Geometry check sheet. Reference: the model listing, model coordinates, mm. Coordinates: 2 decimals unless noted, no trailing zeros. Write each loop counter-clockwise with the first axis right and the second up, starting at its lowest first coordinate (ties: lowest second). Pieces come first, ordered by that corner, then holes. Notation, with made-up numbers: (-15.75, -31.75) -> (31.25, -31.75) arc R21 ccw to (31.25, 3.25) -> close; hole circle Ø7 at (50.25, 47.5). An arc over 180 degrees is marked (long way). One line per question, with ' | ' between items.
Autodesk Inventor part; units mm, degrees
ref_plane "YZ Plane" through (0, 0, 0) normal (1, 0, 0) x (0, 1, 0)
ref_plane "XZ Plane" through (0, 0, 0) normal (0, 1, 0) x (-1, 0, 0)
ref_plane "XY Plane" through (0, 0, 0) normal (0, 0, 1) x (1, 0, 0)
sketch "Sketch1" plane through (0, 0, 0) normal (0, 0, 1) x (1, 0, 0)
  arc A0 (5.0089, -4.6844) -> (-5.0089, -4.6844) centre (0, 0) ccw
  line L0 (0, 0) -> (0, 3.3219)
  line L1 (0, 0) -> (0, -6.858)
  line L2 (4.1269, 0.3611) -> (4.5966, 0.4021)
  line L3 (-4.1269, 0.3611) -> (-4.5966, 0.4021)
  line L4 (-3.0829, -2.3997) -> (-3.5588, -4.3082)
  line L5 (3.0829, -2.3997) -> (3.5588, -4.3082)
  arc A1 (0.8337, 3.4569) -> (-0.8337, 3.4569) centre (0, 0) ccw
  arc A2 (-3.5485, -0.2304) -> (-3.1723, -1.6067) centre (0, 0) ccw
  arc A3 (3.1723, -1.6067) -> (3.5485, -0.2304) centre (0, 0) ccw
  arc A4 (3.5588, -4.3082) -> (5.0089, -4.6844) centre (4.3861, -4.102) ccw
  arc A5 (-5.0089, -4.6844) -> (-3.5588, -4.3082) centre (-4.3861, -4.102) ccw
  arc A6 (4.1269, 0.3611) -> (3.5485, -0.2304) centre (4.1822, -0.2715) ccw
  arc A7 (3.1723, -1.6067) -> (3.0829, -2.3997) centre (4.192, -2.1232) ccw
  arc A8 (-3.5485, -0.2304) -> (-4.1269, 0.3611) centre (-4.1822, -0.2715) ccw
  arc A9 (-3.0829, -2.3997) -> (-3.1723, -1.6067) centre (-4.192, -2.1232) ccw
  arc A10 (4.5966, 0.4021) -> (5.3741, 1.5314) centre (4.5191, 1.2878) ccw
  arc A11 (3.0157, 4.7044) -> (1.3489, 4.3144) centre (2.3718, 3.6998) ccw
  arc A12 (-5.3741, 1.5314) -> (-4.5966, 0.4021) centre (-4.5191, 1.2878) ccw
  arc A13 (-1.3489, 4.3144) -> (-3.0157, 4.7044) centre (-2.3718, 3.6998) ccw
  line L6 (-0.8337, 3.4569) -> (-1.3489, 4.3144)
  line L7 (0.8337, 3.4569) -> (1.3489, 4.3144)
  arc A14 (5.3741, 1.5314) -> (3.0157, 4.7044) centre (0, 0) ccw
  arc A15 (-3.0157, 4.7044) -> (-5.3741, 1.5314) centre (0, 0) ccw
  point P0 (5.5667, 0.487)
  point P1 (-5.5667, 0.487)
  point P2 (-3.7479, -5.1854)
  point P3 (2.9716, -1.9532)
  point P4 (3.7479, -5.1854)
  point P5 (1.4868, 5.1225)
  point P6 (0, 2.4453)
  point P7 (-1.4868, 5.1225)
  point P8 (0, 2.4453)
  point P9 (-2.9716, -1.9532)
  point P10 (-0.8419, 3.4705)
  point P11 (-2.3046, 5.9049)
  point P12 (0.8419, 3.4705)
  point P13 (2.3046, 5.9049)
  dimension "d0" = 13.716
  dimension "d2" = 95
  dimension "d3" = 14
  dimension "d4" = 3.556
  dimension "d5" = 0.8527
  dimension "d6" = 3.556
  dimension "d7" = 14
  dimension "d8" = 1.27
  dimension "d9" = 1.27
  dimension "d10" = 1.778
  dimension "d11" = 31
  dimension "d12" = 2.286
extrude "Extrusion1" add sketch "Sketch1" along normal blind 0.6858
equation "\"d6\" = d4"
equation "\"d7\" = d3"
equation "\"d9\" = d8"
properties material "Steel"
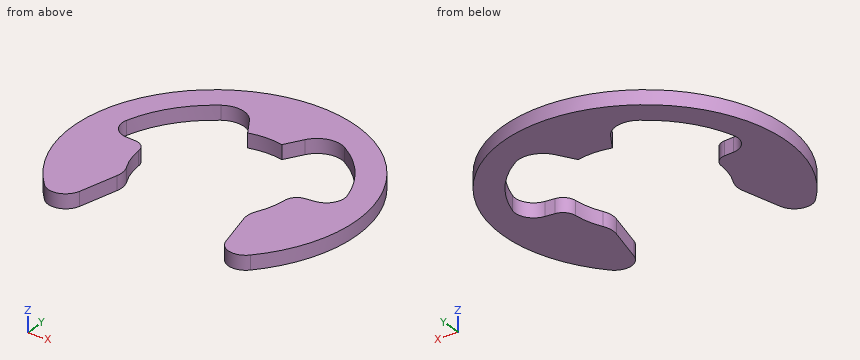
1. Cross-section at C-C on x = 4.75. Record the boundary of the cut face in (y, z).
Worked answers:
outline: (-4.87, 0) -> (0.43, 0) -> (0.43, 0.69) -> (-4.87, 0.69) -> close; (2.94, 0) -> (4.95, 0) -> (4.95, 0.69) -> (2.94, 0.69) -> close
2. Material ranges on line 1 (X direction, y = 1.25, z = 0.1); line 2 (X direction, y = 0, z = 0.15); line 3 (X direction, y = 4.5, z = 0.6), recorded low to high. Write a range as from..to.
Worked answers:
line 1: -6.74..-5.41, 5.41..6.74 | line 2: -6.86..-3.61, 3.61..6.86 | line 3: -5.18..-3.31, -1.49..1.49, 3.31..5.18
3. Go/stop test with a flat-tipped pin: P1, Ø5, axis at x = 2, y = 5, coming from the -Z side. Record where the tip stops, or that it passes through.
Worked answers:
P1: z = 0
4. Cross-section at A-A on z = 0.35. Record the boundary of the cut face in (x, y) (1 decimal), and give its area (3 significant figures).
Worked answers:
outline: (-5.4, 1.5) arc R5.6 cw to (-3, 4.7) arc R1.2 cw to (-1.3, 4.3) -> (-0.8, 3.5) arc R3.6 cw to (0.8, 3.5) -> (1.3, 4.3) arc R1.2 cw to (3, 4.7) arc R5.6 cw to (5.4, 1.5) arc R0.9 cw to (4.6, 0.4) -> (4.1, 0.4) arc R0.6 ccw to (3.5, -0.2) arc R3.6 cw to (3.2, -1.6) arc R1.1 ccw to (3.1, -2.4) -> (3.6, -4.3) arc R0.9 ccw to (5, -4.7) arc R6.9 ccw (long way) to (-5, -4.7) arc R0.9 ccw to (-3.6, -4.3) -> (-3.1, -2.4) arc R1.1 ccw to (-3.2, -1.6) arc R3.6 cw to (-3.5, -0.2) arc R0.6 ccw to (-4.1, 0.4) -> (-4.6, 0.4) arc R0.9 cw to start | area: 61.0 mm²
5. Cross-section at B-B on y = -3.5. Record the boundary of the cut face in (x, z).
Worked answers:
outline: (-5.9, 0) -> (-3.36, 0) -> (-3.36, 0.69) -> (-5.9, 0.69) -> close; (3.36, 0) -> (5.9, 0) -> (5.9, 0.69) -> (3.36, 0.69) -> close
6. Cross-section at D-D on x = 0. Record the boundary of the cut face in (y, z).
Worked answers:
outline: (3.56, 0) -> (6.86, 0) -> (6.86, 0.69) -> (3.56, 0.69) -> close
